Source: three-view drawing plus pictorial views. Frame: mm from the lowest corner of the part. A direction names the side the tool comes from. Give positions to 0.01 mm unless a question says otherwise; leave off trailing zeros. Write each loop counter-clockwise with the first axis right and the second up, starting at its lowest first coordinate (ties: lowest second). Pieces come first, ordered by that corner, then holes.
Q1. Cut plane D-D on z = 37.5. Return the cut outline in (x, y).
Q2. Cut plane A-A on z = 124. Return the cut outline in (x, y), plus the area to 3 significant figures.
Q3. Reachability of the marked faces 4 and 5 from +Z, -Z, +X, -X, +Y, -Y: full face, straight path, thin tool, end or side. Return the list, or none.
Q4. Cut plane B-B on x = 134.5. Return the cut outline in (y, z).
Q5. Cut plane C-C on y = 12.7. Count the separate pieces of the cut face and the enclosed holes in it, plus the area to 3 significant figures.
Q6. Pin query (flat end, axial travel): pin 1 (4 mm diameter, centred on x = 25.4, z = 25.4, fed in from +Y); pin 2 (5.5 mm diameter, centred on y = 12.7, z = 63.5, fed in from +X). Return the tip coordinate at first contact, or that it passes through.
Q7. Line query: L1, parallel to Y at x = 151, z = 190 (1 decimal); L2, parallel to X at y = 35.9, z = 101.6 (1 decimal); L3, parallel to Y at x = 149.95, z = 88.9 (1 decimal). Output: solid intervals per line, ascending.
Q8. Draft query along X for the marked faces 1, 2 and 3. Return one class per face: pulls with the +X half, pulls with the -X half, needs draft (parallel to the pull), parting line crosses it, or undercut.
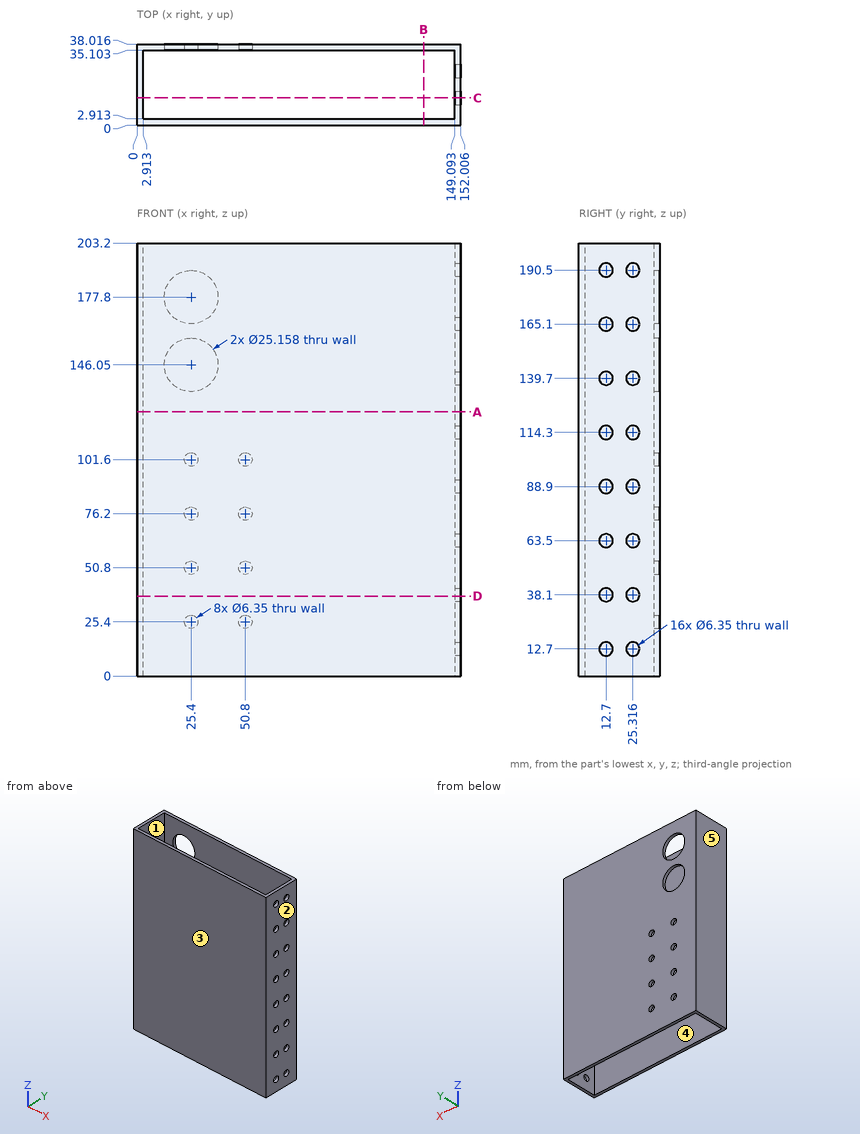
Data:
1. outline: (0, 0) - (152.01, 0) - (152.01, 9.58) - (149.09, 9.58) - (149.09, 2.91) - (2.91, 2.91) - (2.91, 35.1) - (149.09, 35.1) - (149.09, 28.43) - (152.01, 28.43) - (152.01, 38.02) - (0, 38.02) - close; (149.09, 15.82) - (152.01, 15.82) - (152.01, 22.2) - (149.09, 22.2) - close
2. outline: (0, 0) - (152.01, 0) - (152.01, 38.02) - (0, 38.02) - close; hole (2.91, 2.91) - (149.09, 2.91) - (149.09, 35.1) - (2.91, 35.1) - close
2. area: 1,070 mm2
3. face 4: +Z, -Z
3. face 5: +Z, -Z, -X, +Y, -Y
4. outline: (0, 0) - (2.91, 0) - (2.91, 203.2) - (0, 203.2) - close; (35.1, 0) - (38.02, 0) - (38.02, 203.2) - (35.1, 203.2) - close
5. separate pieces: 10
5. enclosed holes: 0
5. area: 1,040 mm2
6. pin 1: stops at y = 2.91
6. pin 2: stops at x = 2.91
7. L1: y = 0 to 9.6, 15.8 to 22.2, 28.5 to 38
7. L2: x = 0 to 22.2, 28.6 to 47.6, 54 to 152
7. L3: y = 0 to 9.5, 15.9 to 22.1, 28.5 to 38
8. face 1: undercut
8. face 2: pulls with the +X half
8. face 3: needs draft
